Verification items for this drawing (mm, ordinates from the low corner). Round coordinates to 2 decimals unless told otherwise and drop trailing zeros. Order: outer loops, then holes, each group sorted by start corner. A loop starts at its lowest first (then second) coordinate and runs counter-clockwise, first axis right, second up.
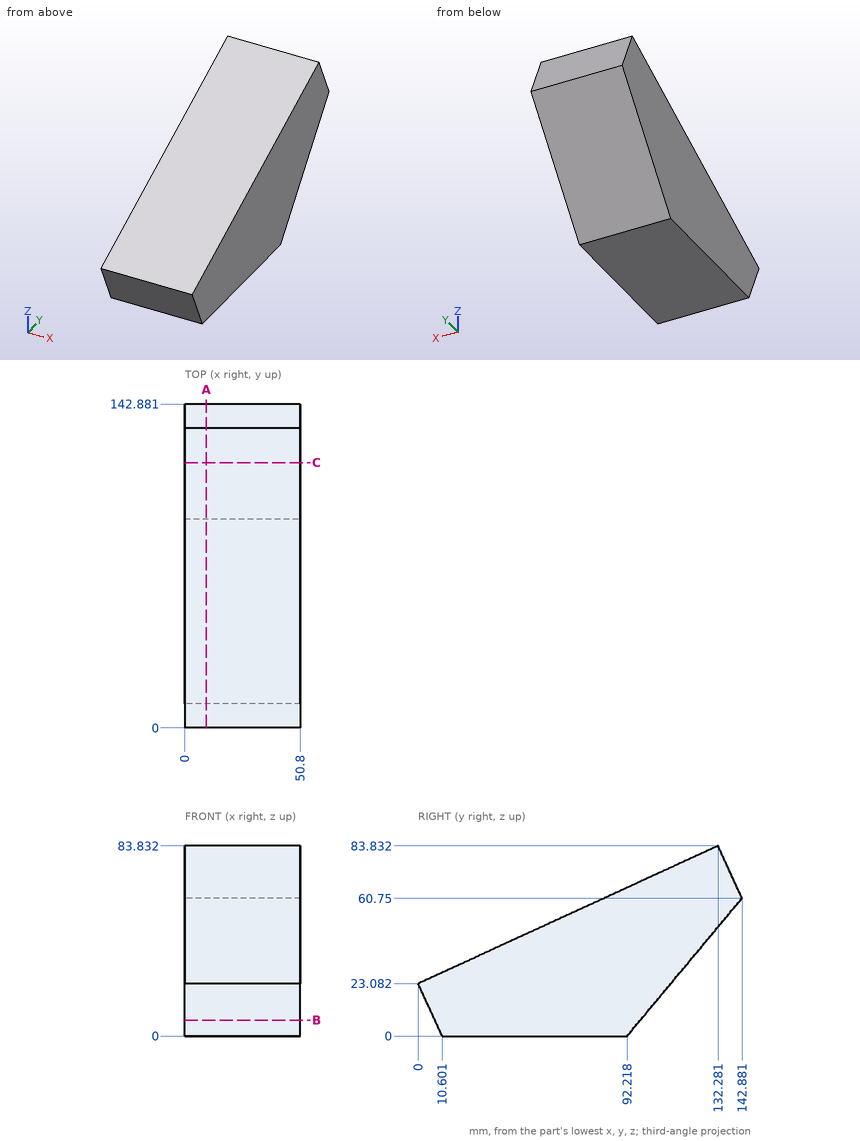
Item 1: Scan lines: line 1 along Y through (x, z) = (5.5, 45.5) (1 decimal); line 2 along Z through (x, y) = (21, 60); line 3 along Y through (x, z) = (8, 42.5) (1 decimal). Record each from-to range of solid material in increasing order.
Answer:
line 1: y = 48.8 to 130.2
line 2: z = 0 to 50.64
line 3: y = 42.3 to 127.7
Item 2: Sectioned sample at A-A (x = 9.5). Record the cut outline in (y, z).
Answer:
outline: (0, 23.08) - (10.6, 0) - (92.22, 0) - (142.88, 60.75) - (132.28, 83.83) - close
Item 3: Sectioned sample at C-C (y = 117). Record the cut outline in (x, z) (1 decimal), and give its area (3 significant figures).
Answer:
outline: (0, 29.7) - (50.8, 29.7) - (50.8, 76.8) - (0, 76.8) - close
area: 2,390 mm2
Item 4: Sectioned sample at B-B (z = 7). Record the cut outline in (x, y) (1 decimal), and give its area (3 significant figures).
Answer:
outline: (0, 7.4) - (50.8, 7.4) - (50.8, 98.1) - (0, 98.1) - close
area: 4,610 mm2
Item 5: Go/stop test with flat-tipped pins: P1, Ø12, axis at x = 41.5, y = 43, coming from the +Z side (1 decimal); P2, Ø5, axis at x = 28.5, z = 74, coming from the -Y side (1 decimal); P3, Ø4, axis at x = 37, y = 36, coming from the +Z side. Record where each tip stops, or that it passes through.
Answer:
P1: stops at z = 45.6
P2: stops at y = 105.4
P3: stops at z = 40.53
